Geometry: final body of the model. Coordinates: model frame, mm. Coordinates: 2 decimals unless noted, no trailing zeros. Order: outer loops, then holes, each group sorted by start corner. A loop starts at its lowest first (then second) coordinate and runs counter-clockwise, first axis right, second up. Notation, with made-up numbers: M 27,79 L 31,79 A12 cw 31,92 Z; hole C 21.25,87.25 d6. An arc over 180 degrees is marked long. Use CSV: the item, a comma, the result in double quotes. Start each with the question number.
Q1. Ray query, probe 1 along Z at (x, y) = (0, 0.5) (3 decimals); probe 2 along X at (y, z) = (-0.8, -2.5) (3 decimals). Return the intervals inside material, ascending.
Q2. First-contact query: P1, Ø12, axis at x = 1.5, z = 0.5, coming from the -Y side. Flat tip, straight axial feed; report the tip coordinate or a pass-through.
Q3. Mould query, pull axis X, two halves, no side actions, for faces 1 (the face through (-15.875, 0, 0)), 2 (the face through (15.875, 0, 0)), 3 (the face through (-1.38, -0.02, 6.2)), 4 (the face through (0, 0, -15.875)). Classes: +X half, -X half, draft (parallel to the pull), parting line (faces both ways), or undercut.
Q4. Section query C-C, the plane y = -0.35. Output: boundary loops of the cut face in (x, z) (3 decimals).
from build123d import *

# Parameters (mm, degrees)
SKETCH1_W           = 31.75
SKETCH1_H           = 31.75
SKETCH1_R           = 6.35
BOSS_EXTRUDE1_DEPTH = 1.5875


with BuildPart() as part:
    # Sketch1 → Boss-Extrude1 (new body, symmetric)
    with BuildSketch(Plane(origin=(0, 0, 0), x_dir=(1, 0, 0), z_dir=(0, 1, 0))):
        Rectangle(SKETCH1_W, SKETCH1_H)
        Circle(SKETCH1_R, mode=Mode.SUBTRACT)
    extrude(amount=BOSS_EXTRUDE1_DEPTH, both=True)


solid = part.part
Responses:
1,probe 1,"z = -15.875 to -6.35, 6.35 to 15.875"
1,probe 2,"x = -15.875 to -5.837, 5.837 to 15.875"
2,P1,"stops at y = -1.59"
3,face 1,"-X half"
3,face 2,"+X half"
3,face 3,"undercut"
3,face 4,"draft"
4,outline,"M -15.875,-15.875 L 15.875,-15.875 L 15.875,15.875 L -15.875,15.875 Z; hole C 0,0 d12.7"
